```python
from build123d import *

# Parameters (mm, degrees)
SKETCH1_W               = 122.684034766
SKETCH1_H               = 85
BOSS_EXTRUDE1_DEPTH     = 58
SKETCH2_W               = 30
SKETCH2_H               = 18.398042608
CUT_EXTRUDE1_DEPTH      = 11.5
CUT_EXTRUDE3_DEPTH      = 5.7
CUT_EXTRUDE3_DEPTH_BACK = 0.0001
SKETCH3_R               = 2
CUT_EXTRUDE4_START      = -5.7
SKETCH5_R               = 2
CUT_EXTRUDE4_DEPTH      = 5.7


with BuildPart() as part:
    # Sketch1 → Boss-Extrude1 (new body)
    # profile 1 of 5: a face of its own
    with BuildSketch(Plane(origin=(0, 0, 0), x_dir=(1, 0, 0), z_dir=(0, 1, 0))):
        Polygon((-68.342017383, -9.5), (-68.342017383, -49.5), (68.342017383, -49.5), (68.342017383, -9.5), (63.842017383, -9.5), (63.842017383, 9.5), (68.342017383, 9.5), (68.342017383, 49.5), (-68.342017383, 49.5), (-68.342017383, 9.5), (-63.842017383, 9.5), (-63.842017383, -9.5), align=None)
        Rectangle(SKETCH1_W, SKETCH1_H, mode=Mode.SUBTRACT)
    # profile 2 of 5: a face of its own
    with BuildSketch(Plane(origin=(0, 0, 0), x_dir=(1, 0, 0), z_dir=(0, 1, 0))):
        Polygon((63.842017383, -9.5), (68.342017383, -9.5), (68.342017383, -7.5), (65.842017383, -7.5), (65.842017383, 7.5), (68.342017383, 7.5), (68.342017383, 9.5), (63.842017383, 9.5), align=None)
    # profile 3 of 5: a face of its own
    with BuildSketch(Plane(origin=(0, 0, 0), x_dir=(1, 0, 0), z_dir=(0, 1, 0))):
        Polygon((68.342017383, -7.5), (68.342017383, -9.5), (72.842017383, -9.5), (72.842017383, 9.5), (68.342017383, 9.5), (68.342017383, 7.5), (70.842017383, 7.5), (70.842017383, -7.5), align=None)
    # profile 4 of 5: a face of its own
    with BuildSketch(Plane(origin=(0, 0, 0), x_dir=(1, 0, 0), z_dir=(0, 1, 0))):
        Polygon((-72.842017383, -9.5), (-68.342017383, -9.5), (-68.342017383, -7.5), (-70.842017383, -7.5), (-70.842017383, 7.5), (-68.342017383, 7.5), (-68.342017383, 9.5), (-72.842017383, 9.5), align=None)
    # profile 5 of 5: a face of its own
    with BuildSketch(Plane(origin=(0, 0, 0), x_dir=(1, 0, 0), z_dir=(0, 1, 0))):
        Polygon((-68.342017383, -7.5), (-68.342017383, -9.5), (-63.842017383, -9.5), (-63.842017383, 9.5), (-68.342017383, 9.5), (-68.342017383, 7.5), (-65.842017383, 7.5), (-65.842017383, -7.5), align=None)
    extrude(amount=BOSS_EXTRUDE1_DEPTH)

    # Sketch2 → Cut-Extrude1 (cut)
    with BuildSketch(Plane.ZY.offset(72.842017383)):
        with Locations((0, 40.800978696)):
            Rectangle(SKETCH2_W, SKETCH2_H)
    extrude(amount=-CUT_EXTRUDE1_DEPTH, mode=Mode.SUBTRACT)

    # Sketch3 → Cut-Extrude3 (cut, two sides: drawn at the far end of the back side and taken through both)
    with BuildSketch(Plane(origin=(0, 0, 0), x_dir=(1, 0, 0), z_dir=(0, 1, 0)).offset(-CUT_EXTRUDE3_DEPTH_BACK)):
        with Locations(Location((64.842017383, -46, 0), (0, 0, 270))):
            Circle(SKETCH3_R)
        with Locations(Location((64.842017383, 46, 0), (0, 0, 90))):
            Circle(SKETCH3_R)
        with Locations(Location((-64.842017383, 46, 0), (0, 0, 270))):
            Circle(SKETCH3_R)
        with Locations(Location((-64.842017383, -46, 0), (0, 0, 90))):
            Circle(SKETCH3_R)
    extrude(amount=CUT_EXTRUDE3_DEPTH + CUT_EXTRUDE3_DEPTH_BACK, mode=Mode.SUBTRACT)

    # Sketch5 → Cut-Extrude4 (cut)
    with BuildSketch(Plane(origin=(0, 58, 0), x_dir=(1, 0, 0), z_dir=(0, 1, 0)).offset(CUT_EXTRUDE4_START)):
        with Locations(Location((-64.842017383, -46, 0), (0, 0, 90))):
            Circle(SKETCH5_R)
        with Locations(Location((64.842017383, -46, 0), (0, 0, 270))):
            Circle(SKETCH5_R)
        with Locations(Location((64.842017383, 19, 0), (0, 0, 270))):
            Circle(SKETCH5_R)
        with Locations(Location((-64.842017383, 19, 0), (0, 0, 90))):
            Circle(SKETCH5_R)
        with Locations(Location((0, 46, 0), (0, 0, 270))):
            Circle(SKETCH5_R)
    extrude(amount=CUT_EXTRUDE4_DEPTH, mode=Mode.SUBTRACT)


solid = part.part
```
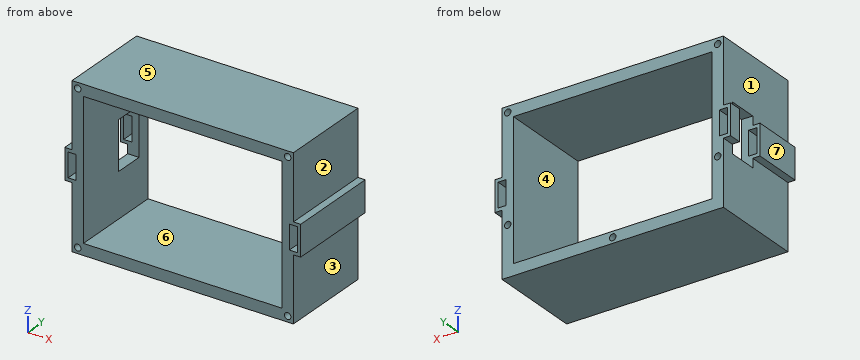
Model file for the job. Use its own axes, mm. Face numbers are marked on the shaded views. A direction names the side the tool comes from. Coordinates: 2 decimals unless noted, no trailing zeros. Order: outer loops, then holes, each group sorted by start corner. A loop starts at its lowest first (then second) coordinate and runs counter-clockwise, first axis right, second up. Notation, with made-up numbers: (-16, 24) - (18, 24) arc R17 ccw to (18, 41) - close; hole circle Ø2 at (-17, 78). An arc over 180 degrees is marked (long way). Return JSON: item names as keys, results as strings. Group by question number.
1) Saw through at A-A, the plane x = 0. Write the cut outline in (y, z).
2) Saw through at C-C, the plane z = -19. Write the cut outline in (x, y).
3) Probe line 1 (X direction, y = 53.6, z = -19); line 2 (X direction, y = 4, z = -46); line 3 (X direction, y = 29.5, z = 1.5). List the from-to ranges inside material, lowest first. Write a range as from..to.
4) Mould opens along X. For the marked faces 4, 5, 6 and 7 say: released by +X, released by -X, zero draft, split by the parting line, or undercut.
5) Saw through at B-B, the plane z = -3.5. Write the cut outline in (x, y), plus the area to 3 significant figures.
6) Tool access for the marked faces 1, 2 and 3: list every direction of +Z, -Z, +X, -X, +Y, -Y with a clear straight run to the whole face (end or side of a thin tool).
7) Flat gauge pins, fed straight in: P1, Ø1.2, axis at x = 0, z = -45.5, coming from the +Y side; P2, Ø10, axis at y = 35, z = -26.5, coming from the +X side; P3, Ø20, axis at y = 28, z = -38, coming from the -X side. Where does each tip first touch, or does it go through?
8) Saw through at D-D, the plane y = 23. Write the cut outline in (x, z), plus the area to 3 significant figures.
Values found:
{
 "1": {"outline": "(0, -49.5) - (58, -49.5) - (58, -48) - (52.3, -48) - (52.3, -44) - (58, -44) - (58, -42.5) - (0, -42.5) - close; (0, 42.5) - (58, 42.5) - (58, 49.5) - (0, 49.5) - close"},
 "2": {"outline": "(-68.34, 0) - (-61.34, 0) - (-61.34, 58) - (-62.84, 58) - (-62.84, 52.3) - (-66.84, 52.3) - (-66.84, 58) - (-68.34, 58) - close; (61.34, 0) - (68.34, 0) - (68.34, 58) - (66.84, 58) - (66.84, 52.3) - (62.84, 52.3) - (62.84, 58) - (61.34, 58) - close"},
 "3": {"line 1": "x = -68.34..-66.84, -62.84..-61.34, 61.34..62.84, 66.84..68.34", "line 2": "x = -68.34..-66.84, -62.84..62.84, 66.84..68.34", "line 3": "x = -72.84..-70.84, -65.84..-61.34, 61.34..65.84, 70.84..72.84"},
 "4": {"face 4": "undercut", "face 5": "zero draft", "face 6": "undercut", "face 7": "released by -X"},
 "5": {"outline": "(-72.84, 0) - (-70.84, 0) - (-70.84, 31.6) - (-72.84, 31.6) - close; (-72.84, 50) - (-70.84, 50) - (-70.84, 58) - (-72.84, 58) - close; (-65.84, 0) - (-61.34, 0) - (-61.34, 31.6) - (-65.84, 31.6) - close; (-65.84, 50) - (-61.34, 50) - (-61.34, 58) - (-65.84, 58) - close; (61.34, 0) - (65.84, 0) - (65.84, 58) - (61.34, 58) - close; (70.84, 0) - (72.84, 0) - (72.84, 58) - (70.84, 58) - close", "area": "634 mm²"},
 "6": {"face 1": "+Z, -X, +Y, -Y", "face 2": "+Z, +X, +Y, -Y", "face 3": "-Z, +X, +Y, -Y"},
 "7": {"P1": "stops at y = 52.3", "P2": "stops at x = 68.34", "P3": "stops at x = -68.34"},
 "8": {"outline": "(-72.84, -9.5) - (-68.34, -9.5) - (-68.34, -49.5) - (68.34, -49.5) - (68.34, -9.5) - (72.84, -9.5) - (72.84, 9.5) - (68.34, 9.5) - (68.34, 49.5) - (-68.34, 49.5) - (-68.34, 9.5) - (-72.84, 9.5) - close; hole (-70.84, -7.5) - (-65.84, -7.5) - (-65.84, 7.5) - (-70.84, 7.5) - close; hole (-61.34, -42.5) - (61.34, -42.5) - (61.34, 42.5) - (-61.34, 42.5) - close; hole (65.84, -7.5) - (70.84, -7.5) - (70.84, 7.5) - (65.84, 7.5) - close", "area": "3,120 mm²"}
}
